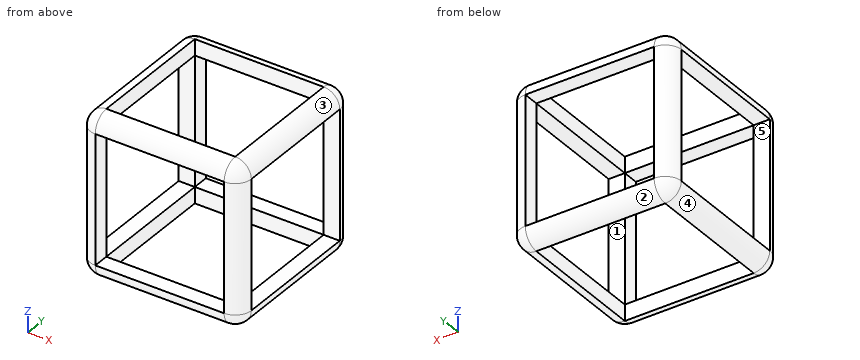
from build123d import *

# Parameters (mm, degrees)
F0_W         = 25.4
F0_H         = 25.4
F1_DEPTH     = 25.4
F2_R         = 2.54
F3_T1_DEPTH  = 20.32
F3_S5_W      = 2.54
F3_S5_H      = 2.54
F3_T6_DEPTH  = 2.54
F3_S11_W     = 2.54
F3_S11_H     = 2.54
F3_T12_DEPTH = 2.54
F4_DEPTH     = 25.401
F5_DEPTH     = 25.401
F6_DEPTH     = 25.401


# Not quite as in the source:
# - a fillet or chamfer that OpenCascade refuses, or shapes differently, is made with other operations: its cross-section is extruded or revolved along the edge and cut away or added


with BuildPart() as f1:
    # F0 (on Front) → F1 (new body)
    with BuildSketch(Plane.XZ):
        with Locations((12.7, -12.7)):
            Rectangle(F0_W, F0_H)
    extrude(amount=F1_DEPTH)

    # F2
    f2_edges = [f1.edges().sort_by_distance(p)[0] for p in [
        (0, 0, -12.7),
        (0, -25.4, -12.7),
        (0, -12.7, -25.4),
        (12.7, 0, -25.4),
        (25.4, 0, -12.7),
        (12.7, 0, 0),
        (0, -12.7, 0),
        (25.4, -12.7, 0),
        (25.4, -12.7, -25.4),
        (25.4, -25.4, -12.7),
        (12.7, -25.4, 0),
    ]]
    fillet(f2_edges, radius=F2_R)

    # F3: fillet of radius 2.54 on 1 edges, made by hand

    # F3_s2 → F3_t1 (cut)
    with BuildSketch(Plane.YZ.offset(2.54)):
        with BuildLine():
            ThreePointArc((-25.4, -22.86), (-24.6560512242, -24.6560512242), (-22.86, -25.4))
            Line((-22.86, -25.4), (-25.4, -25.4))
            Line((-25.4, -25.4), (-25.4, -22.86))
        make_face()
    extrude(amount=F3_T1_DEPTH, mode=Mode.SUBTRACT)


with BuildPart() as f3_tool4:
    # F3_s5 → F3_t6 (new body)
    with BuildSketch(Plane.XZ.offset(22.86)):
        with Locations((1.27, -24.13)):
            Rectangle(F3_S5_W, F3_S5_H)
    extrude(amount=F3_T6_DEPTH)

    # F3_s7 → F3_t8 (revolve, cut)
    with BuildSketch(Plane(origin=(2.54, -22.86, -22.86), x_dir=(0.7071067812, 0, 0.7071067812), z_dir=(0.7071067812, 0, -0.7071067812))):
        with BuildLine():
            ThreePointArc((0, -2.54), (2.54, 0), (0, 2.54))
            Line((0, 2.54), (0, -2.54))
        make_face()
    revolve(axis=Axis((2.54, -22.86, -22.86), (0, -1, 0)), mode=Mode.SUBTRACT)


with BuildPart() as f1_1:
    add(f1.part)

    # F3_t3: cut F3_tool4
    add(f3_tool4.part, mode=Mode.SUBTRACT)


with BuildPart() as f3_tool10:
    # F3_s11 → F3_t12 (new body)
    with BuildSketch(Plane.XZ.offset(22.86)):
        with Locations((24.13, -24.13)):
            Rectangle(F3_S11_W, F3_S11_H)
    extrude(amount=F3_T12_DEPTH)

    # F3_s13 → F3_t14 (revolve, cut)
    with BuildSketch(Plane(origin=(22.86, -22.86, -22.86), x_dir=(-0.7071067812, 0, 0.7071067812), z_dir=(0.7071067812, 0, 0.7071067812))):
        with BuildLine():
            ThreePointArc((0, -2.54), (2.54, 0), (0, 2.54))
            Line((0, 2.54), (0, -2.54))
        make_face()
    revolve(axis=Axis((22.86, -22.86, -22.86), (0, -1, 0)), mode=Mode.SUBTRACT)


with BuildPart() as f1_2:
    add(f1_1.part)

    # F3_t9: cut F3_tool10
    add(f3_tool10.part, mode=Mode.SUBTRACT)

    # F4 (cut, through all): a face of the model
    f4_faces = [f1_2.faces().sort_by_distance(p)[0] for p in [
        (12.7, -12.7, 0),
    ]]
    extrude(f4_faces, amount=-F4_DEPTH, mode=Mode.SUBTRACT)

    # F5 (cut, through all): a face of the model
    f5_faces = [f1_2.faces().sort_by_distance(p)[0] for p in [
        (25.4, -12.7, -12.7),
    ]]
    extrude(f5_faces, amount=-F5_DEPTH, mode=Mode.SUBTRACT)

    # F6 (cut, through all): a face of the model
    f6_faces = [f1_2.faces().sort_by_distance(p)[0] for p in [
        (12.7, 0, -12.7),
    ]]
    extrude(f6_faces, amount=-F6_DEPTH, mode=Mode.SUBTRACT)


solid = f1_2.part
The model under review builds one solid part; all positions refer to its coordinate system, in mm. Face numbers are marked on the shaded views. A direction names the side the tool comes from. Give positions to 0.01 mm unless a question says otherwise; leave off trailing zeros. Loops run counter-clockwise (first coordinate to the right, second up) from the corner with the lowest first, then second, coordinate; pieces in that order, holes last. Notation, with made-up numbers: (12, -18) -> (20, -18) arc R16 cw to (20, -4) -> close; hole circle Ø6 at (-30.5, 18). An arc over 180 degrees is marked (long way). Put each result on its own line as item: value. Start each with the question number.
1. Wall thickness on probe 1 along X at (y, z) = (-23, -13.25); probe 2 along Z at (x, y) = (2.5, -21); probe 3 along Y at (x, z) = (13, -24): over which ranges is each line inside the solid? List them lowest first.
2. Mouldability with a two-part tool opening along Z and no side actions: class the marked faces 1, 2 and 3 as released by +Z, released by -Z, zero draft, split by the parting line, or undercut.
3. We need section C-C on z = -1.25. State the section outline as (x, y) points.
4. We need section B-B on y = -5. State the section outline as (x, z) points.
5. Clearance check with flat-ended pins moving along their axes: P1, Ø0.8, axis at x = 10, z = -25, coming from the +Y side; P2, Ø0.8, axis at x = 0.5, y = -13, coming from the -Z side; P3, Ø1.3, axis at y = -11.5, z = -24.5, coming from the -X side. State where each tip first meets the part, or that it passes through.
6. For the marked faces 4 and 5, list the 3-axis set-ups (+Z, -Z, +X, -X, +Y, -Y) from which the entire face can be reached by the end or side of a thin tool; tool diameter is ignored.
7. We need section A-A on x = 5.75. State the section outline as (y, z) points, then the cut area to 3 significant figures.
Determined:
1. probe 1: 0 to 2.54, 22.86 to 25.4
1. probe 2: -25.4 to -22.86, -2.54 to 0
1. probe 3: -25.13 to -22.86, -2.54 to -0.27
2. face 1: undercut
2. face 2: released by -Z
2. face 3: released by +Z
3. outline: (0.35, -22.86) arc R2.19 ccw to (2.54, -25.05) -> (22.86, -25.05) arc R2.19 ccw to (25.05, -22.86) -> (25.05, -2.54) arc R2.19 ccw to (22.86, -0.35) -> (2.54, -0.35) arc R2.19 ccw to (0.35, -2.54) -> close; hole (2.54, -22.86) -> (22.86, -22.86) -> (22.86, -2.54) -> (2.54, -2.54) -> close
4. outline: (0, -22.86) arc R2.54 ccw to (2.54, -25.4) -> (2.54, -22.86) -> close; (0, -2.54) -> (2.54, -2.54) -> (2.54, 0) arc R2.54 ccw to start; (22.86, -25.4) arc R2.54 ccw to (25.4, -22.86) -> (22.86, -22.86) -> close; (22.86, -2.54) -> (25.4, -2.54) arc R2.54 ccw to (22.86, 0) -> close
5. P1: y = -0.69
5. P2: z = -24.8
5. P3: x = 0.2
6. face 4: -Z, -X, +Y, -Y
6. face 5: +X, -X
7. outline: (-25.4, -22.86) arc R2.54 ccw to (-22.86, -25.4) -> (-22.86, -22.86) -> close; (-25.4, -2.54) -> (-22.86, -2.54) -> (-22.86, 0) arc R2.54 ccw to start; (-2.54, -25.4) arc R2.54 ccw to (0, -22.86) -> (-2.54, -22.86) -> close; (-2.54, -2.54) -> (0, -2.54) arc R2.54 ccw to (-2.54, 0) -> close
7. area: 20.3 mm^2
